from build123d import *

# Parameters (mm, degrees)
BOSS_EXTRUDE1_DEPTH = 102
SKETCH3_R           = 13
BOSS_EXTRUDE3_DEPTH = 2.5
BOSS_EXTRUDE4_DEPTH = 1
FILLET1_R           = 1


with BuildPart() as part:
    # Sketch1 → Revolve1 (revolve)
    with BuildSketch(Plane.XY, mode=Mode.PRIVATE) as revolve1_sk:
        Polygon((0, 0), (7.5, 0), (7.5, 3), (6, 3), (6, 5), (10, 5), (10, 6), (0, 6), align=None)
    revolve(revolve1_sk.sketch.rotate(Axis((0, 6, 0), (0, -1, 0)), 180), axis=Axis((0, 6, 0), (0, -1, 0)))

    # Sketch2 → Boss-Extrude1 (add)
    with BuildSketch(Plane(origin=(0, 6, 0), x_dir=(1, 0, 0), z_dir=(0, 1, 0))):
        with BuildLine():
            Line((-1, 7.891889069), (-1, 1.5))
            ThreePointArc((-1, 1.5), (-1.146446609, 1.146446609), (-1.5, 1))
            Line((-1.5, 1), (-7.304889055, 1))
            ThreePointArc((-7.304889055, 1), (-8.304889055, 0), (-7.304889055, -1))
            Line((-7.304889055, -1), (-1.5, -1))
            ThreePointArc((-1.5, -1), (-1.146446609, -1.146446609), (-1, -1.5))
            Line((-1, -1.5), (-1, -7.891889069))
            ThreePointArc((-1, -7.891889069), (0, -8.891889069), (1, -7.891889069))
            Line((1, -7.891889069), (1, -1.5))
            ThreePointArc((1, -1.5), (1.146446609, -1.146446609), (1.5, -1))
            Line((1.5, -1), (7.304889055, -1))
            ThreePointArc((7.304889055, -1), (8.304889055, 0), (7.304889055, 1))
            Line((7.304889055, 1), (1.5, 1))
            ThreePointArc((1.5, 1), (1.146446609, 1.146446609), (1, 1.5))
            Line((1, 1.5), (1, 7.891889069))
            ThreePointArc((1, 7.891889069), (0, 8.891889069), (-1, 7.891889069))
        make_face()
    extrude(amount=BOSS_EXTRUDE1_DEPTH)

    # Sketch3 → Boss-Extrude3 (add)
    with BuildSketch(Plane(origin=(0, 108, 0), x_dir=(1, 0, 0), z_dir=(0, 1, 0))):
        with Locations(Location((0, 0, 0), (0, 0, 180))):
            Circle(SKETCH3_R)
    extrude(amount=BOSS_EXTRUDE3_DEPTH)

    # Sketch4 → Boss-Extrude4 (add)
    with BuildSketch(Plane(origin=(0, 110.5, 0), x_dir=(1, 0, 0), z_dir=(0, 1, 0))):
        with BuildLine():
            Line((-1.5, 10), (-1.5, -10))
            ThreePointArc((-1.5, -10), (0, -11.5), (1.5, -10))
            Line((1.5, -10), (1.5, 10))
            ThreePointArc((1.5, 10), (0, 11.5), (-1.5, 10))
        make_face()
        with BuildLine():
            Line((-5.7, 8), (-5.7, -8))
            ThreePointArc((-5.7, -8), (-4.2, -9.5), (-2.7, -8))
            Line((-2.7, -8), (-2.7, 8))
            ThreePointArc((-2.7, 8), (-4.2, 9.5), (-5.7, 8))
        make_face()
        with BuildLine():
            Line((-9.9, 6), (-9.9, -6))
            ThreePointArc((-9.9, -6), (-8.4, -7.5), (-6.9, -6))
            Line((-6.9, -6), (-6.9, 6))
            ThreePointArc((-6.9, 6), (-8.4, 7.5), (-9.9, 6))
        make_face()
        with BuildLine():
            Line((6.9, 6), (6.9, -6))
            ThreePointArc((6.9, -6), (8.4, -7.5), (9.9, -6))
            Line((9.9, -6), (9.9, 6))
            ThreePointArc((9.9, 6), (8.4, 7.5), (6.9, 6))
        make_face()
        with BuildLine():
            Line((2.7, 8), (2.7, -8))
            ThreePointArc((2.7, -8), (4.2, -9.5), (5.7, -8))
            Line((5.7, -8), (5.7, 8))
            ThreePointArc((5.7, 8), (4.2, 9.5), (2.7, 8))
        make_face()
    extrude(amount=BOSS_EXTRUDE4_DEPTH)

    # Fillet1
    fillet1_edges = [part.edges().sort_by_distance(p)[0] for p in [
        (9.9, 111.5, 0),
        (8.4, 111.5, 7.5),
        (6.9, 111.5, 0),
        (8.4, 111.5, -7.5),
        (2.7, 111.5, 0),
        (4.2, 111.5, -9.5),
        (5.7, 111.5, 0),
        (4.2, 111.5, 9.5),
        (1.5, 111.5, 0),
        (0, 111.5, 11.5),
        (-1.5, 111.5, 0),
        (0, 111.5, -11.5),
        (-5.7, 111.5, 0),
        (-4.2, 111.5, -9.5),
        (-2.7, 111.5, 0),
        (-4.2, 111.5, 9.5),
        (-6.9, 111.5, 0),
        (-8.4, 111.5, 7.5),
        (-9.9, 111.5, 0),
        (-8.4, 111.5, -7.5),
    ]]
    fillet(fillet1_edges, radius=FILLET1_R - 0.0001)  # a hair under: the kernel refuses the full size


solid = part.part
Could you check a few things on this model? Use its own coordinates, in mm. A direction names the side the tool comes from. Give positions to 0.01 mm unless a question says otherwise; leave off trailing zeros. Loops run counter-clockwise (first coordinate to the right, second up) from the corner with the lowest first, then second, coordinate; pieces in that order, holes last. Notation, with made-up numbers: (-31, -32) -> (-9, -32) arc R25 cw to (-9, -14) -> close; hole circle Ø2 at (15.25, 72). An arc over 180 degrees is marked (long way). Return JSON: item names as keys, results as strings.
Item 1: I'm going to push flat-ended pins straight in: pin 1 (5 mm diameter, centred on y = 44.5, z = -5, fed in from +X); pin 2 (3 mm diameter, centred on y = 60, z = 4, fed in from -X); pin 3 (10 mm diameter, centred on y = 90, z = -1, fed in from +X); pin 4 (6 mm diameter, centred on x = 6, z = -10.5, fed in from +Y). Where does each tip first touch, or does it pass through?
Geometry results:
{"pin 1": "stops at x = 1", "pin 2": "stops at x = -1", "pin 3": "stops at x = 8.3", "pin 4": "stops at y = 111.5"}
Item 2: If we section it at A-A on y = 69: List the corners of the cut face in (x, z) for me.
Geometry results:
{"outline": "(-7.3, -1) -> (-1.5, -1) arc R0.5 cw to (-1, -1.5) -> (-1, -7.89) arc R1 ccw to (1, -7.89) -> (1, -1.5) arc R0.5 cw to (1.5, -1) -> (7.3, -1) arc R1 ccw to (7.3, 1) -> (1.5, 1) arc R0.5 cw to (1, 1.5) -> (1, 7.89) arc R1 ccw to (-1, 7.89) -> (-1, 1.5) arc R0.5 cw to (-1.5, 1) -> (-7.3, 1) arc R1 ccw to start"}
Item 3: I need wall thicknesses on L1, parallel to Y at x = 8.75, z = 2.25; L2, parallel to Y at x = 6.25, z = 5.5; L3, parallel to X at y = 53, z = 7. Which ranges of each line are inside material? Lowest first, please. Write a range as from..to.
Geometry results:
{"L1": "y = 5..6, 108..111.5", "L2": "y = 5..6, 108..110.5", "L3": "x = -1..1"}
Item 4: Which directions (+Z, -Z, +X, -X, +Y, -Y) give clear straight access to the entire face, cutting with the end or side of a thin tool? Please do faces 4 (the cylindrical face through (-4.032, 1.521, -6.324)), 5 (the cylindrical face through (-8.305, 56.286, -0.022)), 6 (the cylindrical face through (-0.02, 56.29, 8.89)), 7 (the flat face through (-1, 56, -5)), 8 (the flat face through (0, 5, 7)).
Geometry results:
{"face 4": "-Y", "face 5": "-X", "face 6": "+Z", "face 7": "-Z, -X", "face 8": "none"}
Item 5: We'd pull the mould along Y, two halves only. Please class faces 1 (the flat face through (0, 0, 0)), 2 (the flat face through (-2, 3, -6)), 3 (the flat face through (2, 110.5, -1)): +Y half, -Y half, draft (parallel to the pull), parting line (faces both ways), or undercut.
Geometry results:
{"face 1": "-Y half", "face 2": "undercut", "face 3": "+Y half"}
